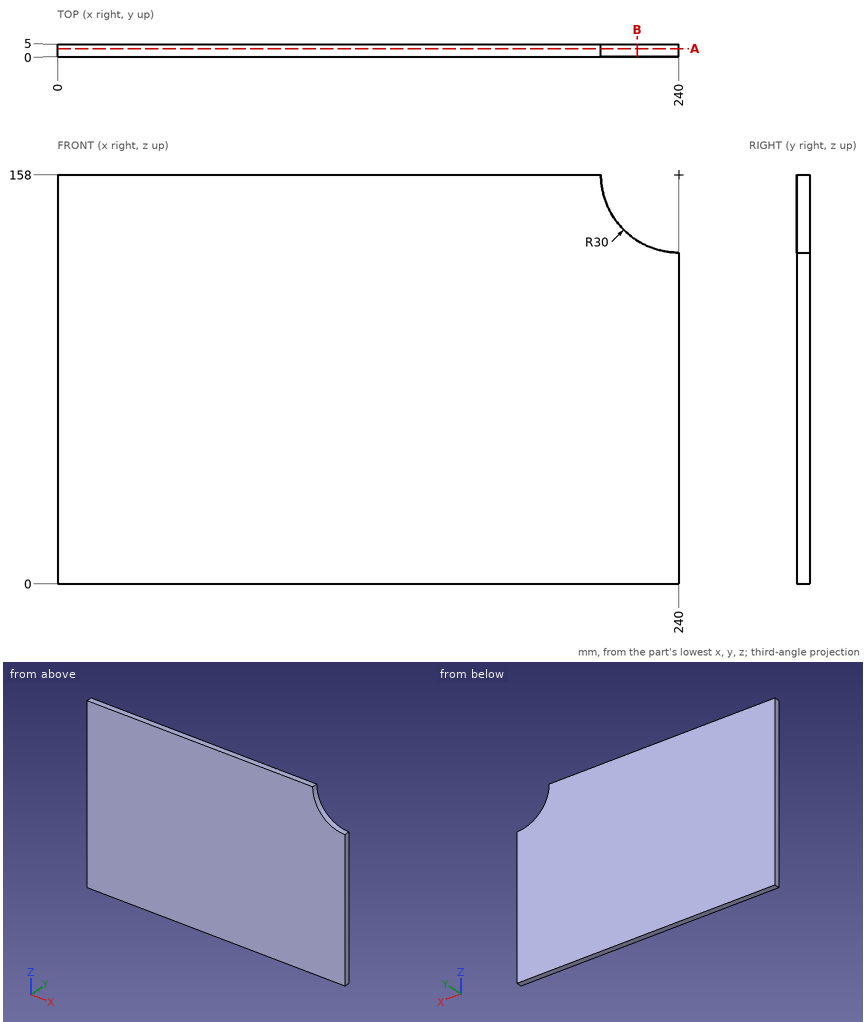
Design review of the part shown in the three views and the two pictorial views. Dimensions are in mm from the part's minimum x, y and z. Round coordinates to 2 decimals unless told otherwise and drop trailing zeros. Write each loop counter-clockwise with the first axis right and the second up, starting at its lowest first coordinate (ties: lowest second). Pieces come first, ordered by that corner, then holes. Notation, with made-up numbers: (-10.5, 36) - (-6.5, 36) arc R19 cw to (-6.5, 66) - close; hole circle Ø1 at (41.25, 83.5). An arc over 180 degrees is marked (long way). Return JSON: item names as keys, results as strings. Group by question number.
Item 1: We need section B-B on x = 224. Write out the cut boundary in (y, z).
Item 2: We need section A-A on y = 3.2. Write out the cut boundary in (x, z).
Item 3: For probe 1 along X at (y, z) = (0.35, 145); probe 2 along Z at (x, y) = (229, 4.4); probe 3 along X at (y, z) = (4.75, 141), list the stretches that pass through material, from the lowest coordinate up. Write a range as [from, to].
Item 4: Insertion check: P1, Ø1.5, axis at x = 48.5, z = 45.5, coming from the -Y side; P2, Ø1.5, axis at y = 4, z = 140, coming from the +X side. Each pin has a flat end and moves straight along its axis. Give the tip position at first contact, or say it passes through.
Model answer:
{
 "1": {"outline": "(0, 0) - (5, 0) - (5, 132.62) - (0, 132.62) - close"},
 "2": {"outline": "(0, 0) - (240, 0) - (240, 128) arc R30 cw to (210, 158) - (0, 158) - close"},
 "3": {"probe 1": "x = [0, 212.96]", "probe 2": "z = [0, 130.09]", "probe 3": "x = [0, 215.28]"},
 "4": {"P1": "stops at y = 0", "P2": "stops at x = 216.58"}
}
